Read the model definition and answer for the solid it produces. Units are mm, in the model's axes. Coordinates: 2 decimals unless noted, no trailing zeros. Write each loop counter-clockwise with the first axis right and the second up, starting at its lowest first coordinate (ties: lowest second). Pieces come first, ordered by that corner, then holes. Notation, with made-up numbers: (4, -17.75) -> (13, -17.75) arc R24 cw to (13, 20.25) -> close; hole circle Ø9 at (-13, -3). An arc over 180 degrees is marked (long way). Answer in a Markdown table with one row per item. Add a question column.
Item 1: Given pin 1 Ø6 at (x, y) = (14.605, 14.605) entering from -Z (1 decimal), flat-ended and moving along its own axis, determine where the tip first touches the part or whether it passes through.
Item 2: Straight lines are drawn through the part: line 1 (Y direction, x = 0, z = 0.2); line 2 (Y direction, x = -17, z = -0.25); line 3 (Y direction, x = -15, z = 0.05). For each, find the intervals that lie inside material, in ascending order. Write a range as from..to.
Item 3: Section A-A on x = 0 is taken. Write down the section's boundary in (y, z), then the cut area to 3 significant figures.
Item 4: Section C-C on y = 13 is taken. Write down the section's boundary in (x, z).
Item 5: Section D-D on z = -0.1 is taken. Write down the section's boundary in (x, y) (3 decimals).
```python
from build123d import *

# Parameters (mm, degrees)
SKETCH1_W                = 41.402
SKETCH1_H                = 41.402
BOSS_EXTRUDE1_DEPTH      = 0.499999
BOSS_EXTRUDE1_DEPTH_BACK = 0.499999
SKETCH3_R                = 16.51
CUT_EXTRUDE1_DEPTH       = 1.999998
SKETCH6_R                = 3.302
CUT_EXTRUDE2_DEPTH       = 1.999998


with BuildPart() as part:
    # Sketch1 → Boss-Extrude1 (new body, two sides)
    with BuildSketch(Plane.XY) as boss_extrude1_sk:
        Rectangle(SKETCH1_W, SKETCH1_H)
    extrude(amount=BOSS_EXTRUDE1_DEPTH)
    extrude(boss_extrude1_sk.sketch, amount=-BOSS_EXTRUDE1_DEPTH_BACK)

    # Sketch3 → Cut-Extrude1 (cut, through all)
    with BuildSketch(Plane.XY.offset(0.499999)):
        Circle(SKETCH3_R)
    extrude(amount=-CUT_EXTRUDE1_DEPTH, mode=Mode.SUBTRACT)

    # Sketch6 → Cut-Extrude2 (cut, through all)
    with BuildSketch(Plane.XY.offset(0.499999)):
        with Locations((-14.605, 14.605)):
            Circle(SKETCH6_R)
        with Locations((14.605, 14.605)):
            Circle(SKETCH6_R)
    cut_extrude2 = extrude(amount=-CUT_EXTRUDE2_DEPTH, mode=Mode.SUBTRACT)

    # Mirror1: Cut-Extrude2 across plane
    add(cut_extrude2.mirror(Plane.ZX), mode=Mode.SUBTRACT)


solid = part.part
```
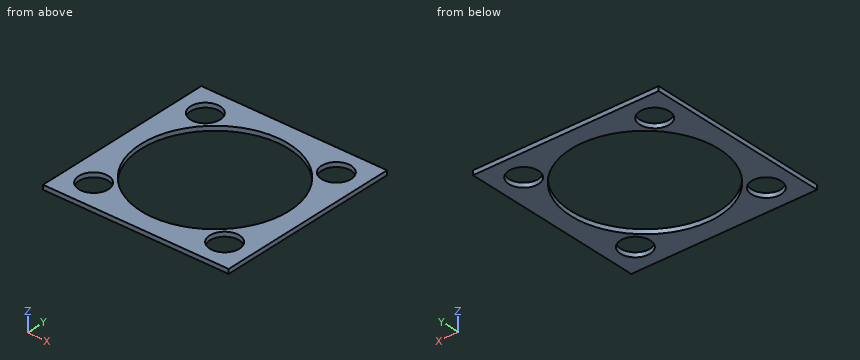
Results below:
| question | item | result |
|---|---|---|
| 1 | pin 1 | passes through |
| 2 | line 1 | y = -20.7..-16.51, 16.51..20.7 |
| 2 | line 2 | y = -20.7..-16.88, -12.33..12.33, 16.88..20.7 |
| 2 | line 3 | y = -20.7..-17.88, -11.33..-6.9, 6.9..11.33, 17.88..20.7 |
| 3 | outline | (-20.7, -0.5) -> (-16.51, -0.5) -> (-16.51, 0.5) -> (-20.7, 0.5) -> close; (16.51, -0.5) -> (20.7, -0.5) -> (20.7, 0.5) -> (16.51, 0.5) -> close |
| 3 | area | 8.38 mm2 |
| 4 | outline | (-20.7, -0.5) -> (-17.49, -0.5) -> (-17.49, 0.5) -> (-20.7, 0.5) -> close; (-11.72, -0.5) -> (-10.18, -0.5) -> (-10.18, 0.5) -> (-11.72, 0.5) -> close; (10.18, -0.5) -> (11.72, -0.5) -> (11.72, 0.5) -> (10.18, 0.5) -> close; (17.49, -0.5) -> (20.7, -0.5) -> (20.7, 0.5) -> (17.49, 0.5) -> close |
| 5 | outline | (-20.701, -20.701) -> (20.701, -20.701) -> (20.701, 20.701) -> (-20.701, 20.701) -> close; hole circle Ø6.604 at (-14.605, -14.605); hole circle Ø6.604 at (-14.605, 14.605); hole circle Ø33.02 at (0, 0); hole circle Ø6.604 at (14.605, -14.605); hole circle Ø6.604 at (14.605, 14.605) |
